```python
from build123d import *

# Parameters (mm, degrees)
F0_W           = 40
F0_H           = 27
F1_DEPTH       = 150
F2_W           = 15.5
F2_H           = 3.5
F3_DEPTH       = 20
F5_W           = 35
F5_H           = 35
F5_R           = 8.5
F6_DEPTH       = 25
F4_R           = 8.5
F7_DEPTH       = 25
F8_R           = 5.5
F9_DEPTH       = 52.001
F10_S5_R       = 8.5
F10_T6_DEPTH   = 14
F11_R          = 5
F13_DEPTH      = 150
F14_T1_DEPTH   = 65
F14_T3_DEPTH   = 37.5
F15_R          = 2
F16_R          = 2.5
F17_DEPTH      = 20.001
F17_DEPTH_BACK = 25
F18_SIZE       = 3


# Not quite as in the source:
# - a fillet or chamfer that OpenCascade refuses, or shapes differently, is made with other operations: its cross-section is extruded or revolved along the edge and cut away or added


with BuildPart() as f1:
    # F0 (on Front) → F1 (new body)
    with BuildSketch(Plane.XZ):
        Rectangle(F0_W, F0_H)
    extrude(amount=F1_DEPTH)

    # F2 (on face) → F3 (cut)
    with BuildSketch(Plane.XY.offset(13.5)):
        with Locations((0, -1.75)):
            Rectangle(F2_W, F2_H)
        Polygon((-7.75, -3.5), (-10, -3.5), (-10, -35.5), (10, -35.5), (10, -3.5), (7.75, -3.5), align=None)
        Polygon((-10, -146.5), (-7.75, -146.5), (7.75, -146.5), (10, -146.5), (10, -114.5), (-10, -114.5), align=None)
        with Locations((0, -148.25)):
            Rectangle(F2_W, F2_H)
    extrude(amount=-F3_DEPTH, mode=Mode.SUBTRACT)

    # F5 (on face) → F6 (join)
    with BuildSketch(Plane(origin=(0, 0, -13.5), x_dir=(1, 0, 0), z_dir=(0, 0, -1))):
        with Locations((0, 75)):
            Rectangle(F5_W, F5_H)
        with Locations((0, 75)):
            Circle(F5_R, mode=Mode.SUBTRACT)
    extrude(amount=F6_DEPTH)

    # F4 (on face) → F7 (cut)
    with BuildSketch(Plane(origin=(0, 0, -13.5), x_dir=(1, 0, 0), z_dir=(0, 0, -1))):
        with Locations((0, 75)):
            Circle(F4_R)
    extrude(amount=-F7_DEPTH, mode=Mode.SUBTRACT)

    # F8 (on face) → F9 (cut, through all)
    with BuildSketch(Plane.XY.offset(13.5)):
        with Locations((0, -75)):
            Circle(F8_R)
    extrude(amount=-F9_DEPTH, mode=Mode.SUBTRACT)

    # F10: chamfer of 3 on 1 edges, made by hand


with BuildPart() as f10_tool2:
    # F10_s3 → F10_t4 (revolve)
    with BuildSketch(Plane.XZ.offset(75)):
        Polygon((5.5, 14.5), (8.5, 11.5), (5.5, 11.5), align=None)
    revolve(axis=Axis((0, -75, 11.5), (0, 0, 1)))

    # F10_s5 → F10_t6 (intersect, symmetric)
    with BuildSketch(Plane.XY.offset(13)):
        with Locations((0, -75)):
            Circle(F10_S5_R)
    extrude(amount=F10_T6_DEPTH, both=True, mode=Mode.INTERSECT)


with BuildPart() as f1_1:
    add(f1.part)

    # F10_t1: cut F10_tool2
    add(f10_tool2.part, mode=Mode.SUBTRACT)

    # F11
    f11_edges = [f1_1.edges().sort_by_distance(p)[0] for p in [
        (-8.5, -75, 11.5),
    ]]
    fillet(f11_edges, radius=F11_R)

    # F12 (on Front) → F13 (join, through all)
    with BuildSketch(Plane.XZ):
        Polygon((10.7683869545, 26.5), (15.5, 13.5), (20, 13.5), (20, 26.5), align=None)
        Polygon((-20, 26.5), (-20, 13.5), (-15.5, 13.5), (-10.7683869545, 26.5), align=None)
    extrude(amount=F13_DEPTH)

    # F14: fillet of radius 5 on 8 edges, made by hand

    # F14_s2 → F14_t1 (cut)
    with BuildSketch(Plane.XY.offset(-26)):
        with BuildLine():
            ThreePointArc((-20, -145), (-18.5355339059, -148.5355339059), (-15, -150))
            Line((-15, -150), (-20, -150))
            Line((-20, -150), (-20, -145))
        make_face()
        with BuildLine():
            ThreePointArc((20, -145), (18.5355339059, -148.5355339059), (15, -150))
            Line((15, -150), (20, -150))
            Line((20, -150), (20, -145))
        make_face()
        with BuildLine():
            ThreePointArc((20, -5), (18.5355339059, -1.4644660941), (15, 0))
            Line((15, 0), (20, 0))
            Line((20, 0), (20, -5))
        make_face()
        with BuildLine():
            ThreePointArc((-20, -5), (-18.5355339059, -1.4644660941), (-15, 0))
            Line((-15, 0), (-20, 0))
            Line((-20, 0), (-20, -5))
        make_face()
    extrude(amount=F14_T1_DEPTH, mode=Mode.SUBTRACT)

    # F14_s4 → F14_t3 (cut)
    with BuildSketch(Plane.XY.offset(-51)):
        with BuildLine():
            ThreePointArc((12.5, -57.5), (16.0355339059, -58.9644660941), (17.5, -62.5))
            Line((17.5, -62.5), (17.5, -57.5))
            Line((17.5, -57.5), (12.5, -57.5))
        make_face()
        with BuildLine():
            ThreePointArc((12.5, -92.5), (16.0355339059, -91.0355339059), (17.5, -87.5))
            Line((17.5, -87.5), (17.5, -92.5))
            Line((17.5, -92.5), (12.5, -92.5))
        make_face()
        with BuildLine():
            ThreePointArc((-17.5, -62.5), (-16.0355339059, -58.9644660941), (-12.5, -57.5))
            Line((-12.5, -57.5), (-17.5, -57.5))
            Line((-17.5, -57.5), (-17.5, -62.5))
        make_face()
        with BuildLine():
            ThreePointArc((-12.5, -92.5), (-16.0355339059, -91.0355339059), (-17.5, -87.5))
            Line((-17.5, -87.5), (-17.5, -92.5))
            Line((-17.5, -92.5), (-12.5, -92.5))
        make_face()
    extrude(amount=F14_T3_DEPTH, mode=Mode.SUBTRACT)

    # F15
    f15_edges = [f1_1.edges().sort_by_distance(p)[0] for p in [
        (-12.884193, -150, 26.5),
        (12.884193, -150, 26.5),
    ]]
    fillet(f15_edges, radius=F15_R)

    # F16 (on Right) → F17 (cut, two sides)
    with BuildSketch(Plane.YZ) as f17_sk:
        with Locations((-100, 1.5)):
            Circle(F16_R)
        with Locations((-50, 1.5)):
            Circle(F16_R)
    extrude(amount=-F17_DEPTH, mode=Mode.SUBTRACT)
    extrude(f17_sk.sketch, amount=F17_DEPTH_BACK, mode=Mode.SUBTRACT)

    # F18
    f18_edges = [f1_1.edges().sort_by_distance(p)[0] for p in [
        (-20, -52.5, 1.5),
        (-20, -102.5, 1.5),
    ]]
    chamfer(f18_edges, length=F18_SIZE)


solid = f1_1.part
```
Work out the finished part from the listing and answer in its coordinate system (mm). A direction names the side the tool comes from. Give positions to 0.01 mm unless a question says otherwise; leave off trailing zeros. Write each loop counter-clockwise with the first axis right and the second up, starting at its lowest first coordinate (ties: lowest second). Pieces come first, ordered by that corner, then holes. Notation, with made-up numbers: (81, 4) - (108, 4) arc R27 cw to (108, 37) - close; hole circle Ø7 at (11, 66). An arc over 180 degrees is marked (long way). Use one line per item in the form item = value.
1. Determine the mould class of faces 1 (the face through (1.76, -47.69, 0.54)), 2 (the face through (16, -91.07, -26.18)), 3 (the face through (-7.75, -2, 4)) for opening direction X: released by +X, released by -X, zero draft, split by the parting line, or undercut.
Filled in:
face_1 = zero draft
face_2 = released by +X
face_3 = undercut
2. For faces 4 (the face through (0, -35.5, 4)), 5 (the face through (-13.167, -73.95, 19.909)), 6 (the face through (4.57, -82.167, -14.2)), 7 (the face through (7.75, -148, 4)), determine the directions among +Z, -Z, +X, -X, +Y, -Y from which every point of the face is accessible in a straight line to the end or side of a thin tool.
Filled in:
face_4 = +Z
face_5 = +Y, -Y
face_6 = -Z
face_7 = +Z, -Y
3. A cutting plane is placed at D-D (y = -16). Write down the section's boundary in (x, z).
Filled in:
outline = (-20, -13.5) - (20, -13.5) - (20, 24.5) arc R2 ccw to (18, 26.5) - (10.77, 26.5) - (15.5, 13.5) - (10, 13.5) - (10, -6.5) - (-10, -6.5) - (-10, 13.5) - (-15.5, 13.5) - (-10.77, 26.5) - (-18, 26.5) arc R2 ccw to (-20, 24.5) - close
4. Each of these flat-tipped pins is pushed along its axis until it touches: pin 1 Ø2 at (y, z) = (-67, -21.5) entering from +X; pin 2 Ø4 at (y, z) = (-2.5, 1.5) entering from -X; pin 3 Ø1 at (x, y) = (13, -38) entering from -Z. Where does it stop, or does it pass through?
Filled in:
pin_1 = 17.5
pin_2 = -19.97
pin_3 = -13.5
5. A cutting plane is placed at C-C (y = -100). Write down the section's boundary in (x, z), and give its area (3 significant figures).
Filled in:
outline = (-20, -13.5) - (20, -13.5) - (20, -1) - (-17, -1) - (-20, -4) - close; (-20, 7) - (-17, 4) - (20, 4) - (20, 24.5) arc R2 ccw to (18, 26.5) - (10.77, 26.5) - (15.5, 13.5) - (-15.5, 13.5) - (-10.77, 26.5) - (-18, 26.5) arc R2 ccw to (-20, 24.5) - close
area = 1,050 mm^2
6. A cutting plane is placed at B-B (x = 0). State how many separate pieces and enclosed holes the cut face has, and give its area (3 significant figures).
Filled in:
separate_pieces = 2
enclosed_holes = 2
area = 2,590 mm^2
7. Consider L1, parallel to Y at x = 0, z = -14; L2, parallel to Y at x = 2, z = 1.5; L3, parallel to Y at x = 0, z = 1.5. Determine where each line is inside the solid, lowest interval first.
Filled in:
L1 = -92.5 to -83.5, -66.5 to -57.5
L2 = -114.5 to -102.5, -97.5 to -83.26, -66.74 to -52.5, -47.5 to -35.5
L3 = -114.5 to -102.5, -97.5 to -83.5, -66.5 to -52.5, -47.5 to -35.5
8. A cutting plane is placed at A-A (z = -10.5). Write down the section's boundary in (x, y).
Filled in:
outline = (-20, -145) arc R5 ccw to (-15, -150) - (15, -150) arc R5 ccw to (20, -145) - (20, -5) arc R5 ccw to (15, 0) - (-15, 0) arc R5 ccw to (-20, -5) - close; hole circle Ø17 at (0, -75)
